Input: part model. Units: mm. Frame: model coordinates. A direction names the side the tool comes from. Round coordinates to 2 decimals unless told otherwise and drop trailing zeros. Loops run counter-clockwise (first coordinate to the right, second up) from the corner with the lowest first, then second, coordinate; pieces in that order, holes last. Notation, with made-up numbers: M 37.25,-19 L 41.25,-19 A13 cw 41.25,-7 Z; hole C 79,27 d5. An arc over 180 degrees is marked long. Put each result on its own line as item: value. Start each with the question number.
1) Section D-D on z = 29.5. Output: boundary loops of the cut face in (x, y), plus the area to 3 significant figures.
2) Section B-B on y = 5. Output: boundary loops of the cut face in (x, z), plus the area to 3 significant figures.
3) Line query: probe 1 along Z at (x, y) = (0, 1.5); probe 2 along Y at (x, z) = (-12.5, 57.5). Output: solid intervals per line, ascending.
4) Reachability of faces 5 (the face through (25.4, 5, 22)), 6 (the face through (-6, 6.35, 35)) from +Z, -Z, +X, -X, +Y, -Y: full face, straight path, thin tool, end or side. Return the list, or none.
5) Pin query (flat end, axial travel): pin 1 (4 mm diameter, centred on x = 16, y = 27, fed in from +Z); pin 2 (10 mm diameter, centred on x = 0, z = 39.45, fed in from -Y). Return the tip coordinate at first contact, or that it passes through.
6) Section C-C on z = 36. Output: boundary loops of the cut face in (x, y).
7) Section A-A on x = 0. Output: boundary loops of the cut face in (y, z).
8) Draft query along X for faces 1 (the face through (0.07, 36.27, 3.13)), 2 (the face through (-25.4, 5, 22)), 3 (the face through (0, 0, 32)), 4 (the face through (2.93, 3.131, 33.813)). Return one class per face: +X half, -X half, draft (parallel to the pull), parting line (faces both ways), or undercut.
Autodesk Inventor part; units mm, degrees
ref_plane "YZ Plane" through (0, 0, 0) normal (1, 0, 0) x (0, 1, 0)
ref_plane "XZ Plane" through (0, 0, 0) normal (0, 1, 0) x (-1, 0, 0)
ref_plane "XY Plane" through (0, 0, 0) normal (0, 0, 1) x (1, 0, 0)
sketch "Sketch1" plane through (0, 0, 0) normal (1, 0, 0) x (0, 1, 0)
  line L0 (0, 0) -> (39.4462, 0)
  line L1 (39.4462, 0) -> (39.4462, 6.35)
  line L2 (39.4462, 6.35) -> (6.35, 6.35)
  line L3 (6.35, 6.35) -> (6.35, 63.5)
  line L4 (6.35, 63.5) -> (0, 63.5)
  line L5 (0, 63.5) -> (0, 0)
  dimension "d0" = 6.35
  dimension "d1" = 6.35
  dimension "d4" = 33.0962
  dimension "d11" = 63.5
extrude "Extrusion1" add sketch "Sketch1" along normal mid plane 50.8
sketch "Sketch2" plane through (25.4, 39.4462, 0) normal (0, 0, -1) x (-1, 0, 0)
  line L0 (50.8, 0) -> (0, 0)
  arc A0 (22.225, 0) -> (28.575, 0) centre (25.4, 0) ccw
  line L1 (28.575, 0) -> (22.225, 0)
  point P0 (25.4, -39.4462)
  dimension "d5" = 6.35
extrude "Extrusion2" cut sketch "Sketch2" against normal through all
sketch "Sketch4" plane through (-25.4, 0, 0) normal (0, -1, 0) x (1, 0, 0)
  line L0 (25.4, 0) -> (25.4, 63.5) construction
  line L1 (0, 63.5) -> (50.8, 63.5) construction
  line L2 (0, 39.4462) -> (50.8, 39.4462) construction
  line L3 (50.8, 0) -> (0, 0) construction
  circle A0 centre (25.4, 39.4462) radius 6.35
  dimension "d12" = 39.4462
  dimension "d13" = 12.7
extrude "Extrusion4" cut sketch "Sketch4" against normal through all
properties part number "Angle Bracket for Bevel Gearbox"
Geometry results:
1. outline: M -25.4,0 L 25.4,0 L 25.4,6.35 L -25.4,6.35 Z
1. area: 323 mm²
2. outline: M -25.4,0 L 25.4,0 L 25.4,63.5 L -25.4,63.5 Z; hole C 0,39.45 d12.7
2. area: 3,100 mm²
3. probe 1: z = 0 to 33.1, 45.8 to 63.5
3. probe 2: y = 0 to 6.35
4. face 5: +Z, -Z, +X, +Y, -Y
4. face 6: +Z, +X, -X, +Y
5. pin 1: stops at z = 6.35
5. pin 2: passes through
6. outline: M -25.4,0 L -5.33,0 L -5.33,6.35 L -25.4,6.35 Z; M 5.33,0 L 25.4,0 L 25.4,6.35 L 5.33,6.35 Z
7. outline: M 0,0 L 36.27,0 L 36.27,6.35 L 6.35,6.35 L 6.35,33.1 L 0,33.1 Z; M 0,45.8 L 6.35,45.8 L 6.35,63.5 L 0,63.5 Z
8. face 1: undercut
8. face 2: -X half
8. face 3: draft
8. face 4: undercut
